Build history of the part. All positions in model axes, mm. Face numbers are marked on the shaded views. A direction names the side the tool comes from. Round coordinates to 2 decimals unless told otherwise and drop trailing zeros. Loops run counter-clockwise (first coordinate to the right, second up) from the corner with the lowest first, then second, coordinate; pieces in that order, holes last. Notation, with made-up numbers: M -27,4.25 L 0,4.25 A16 ccw 0,31.25 Z; hole C 63,-30.75 d8. An arc over 180 degrees is marked long. Use one line per item in the form item = value. Start each with the question number.
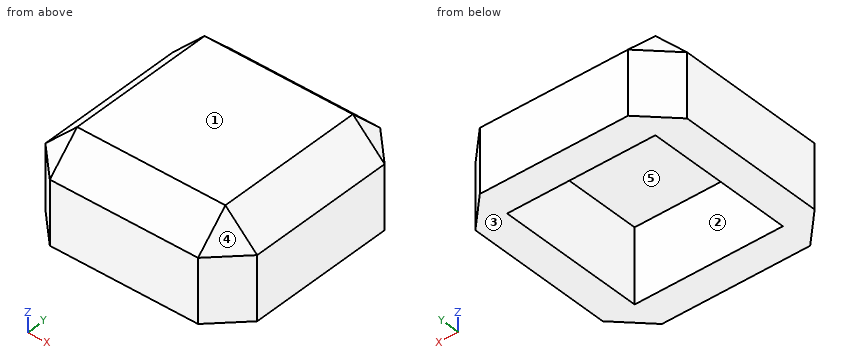
```python
from build123d import *

# Parameters (mm, degrees)
F0_W     = 10
F0_H     = 10
F0_W_2   = 7
F0_H_2   = 7
F1_DEPTH = 1
F2_DEPTH = 3.5
F3_SIZE  = 1.5


with BuildPart() as f1:
    # F0 (on Top) → F1 (new body)
    with BuildSketch(Plane.XY):
        Rectangle(F0_W, F0_H)
        Rectangle(F0_W_2, F0_H_2, mode=Mode.SUBTRACT)
        Rectangle(F0_W_2, F0_H_2)
    extrude(amount=F1_DEPTH)

    # F0 (on Top) → F2 (join)
    with BuildSketch(Plane.XY):
        Rectangle(F0_W, F0_H)
        Rectangle(F0_W_2, F0_H_2, mode=Mode.SUBTRACT)
    extrude(amount=-F2_DEPTH)

    # F3
    f3_edges = [f1.edges().sort_by_distance(p)[0] for p in [
        (5, -5, -1.25),
        (-5, -5, -1.25),
        (-5, 5, -1.25),
        (5, 5, -1.25),
        (0, -5, 1),
        (0, 5, 1),
        (-5, 0, 1),
        (5, 0, 1),
    ]]
    chamfer(f3_edges, length=F3_SIZE)


solid = f1.part
```
Q1. Saw through at B-B (z = 0.35). Give the cut face in (x, y), and give its area (3 significant figures).
Q2. Pull direction Z, two halves, no side cores. Call the marked faces 1, 2 and 3: pulls with the +Z half, pulls with the -Z half, needs draft (parallel to the pull), parting line crosses it, or undercut.
Q3. Tool access for the marked faces 4 and 5: list every direction of +Z, -Z, +X, -X, +Y, -Y with a clear straight run to the whole face (end or side of a thin tool).
Q4. Saw through at D-D (z = -1.05). Give the cut face in (x, y), and give its area (3 significant figures).
Q5. Saw through at C-C (x = 3.75). Give the cut face in (y, z).
Q6. Drop a flat-ended pin along its axis: P1, Ø1.5, axis at x = 1, y = 0, coming from the -Z side. Give the stop position or say it passes through.
Q7. Wall check: probe 1 along X at (y, z) = (0.25, -2.15); probe 2 along Z at (x, y) = (3.25, 2.5). Give the ranges that are in metal, low to high.
Q8. Saw through at A-A (y = 1). Give the cut face in (x, z).
Filled in:
q1.outline = M -4.15,-3.5 L -3.5,-4.15 L 3.5,-4.15 L 4.15,-3.5 L 4.15,3.5 L 3.5,4.15 L -3.5,4.15 L -4.15,3.5 Z
q1.area = 68.0 mm²
q2.face_1 = pulls with the +Z half
q2.face_2 = needs draft
q2.face_3 = pulls with the -Z half
q3.face_4 = +Z, +X, -Y
q3.face_5 = -Z
q4.outline = M -5,-3.5 L -3.5,-5 L 3.5,-5 L 5,-3.5 L 5,3.5 L 3.5,5 L -3.5,5 L -5,3.5 Z; hole M -3.5,-3.5 L 3.5,-3.5 L 3.5,3.5 L -3.5,3.5 Z
q4.area = 46.5 mm²
q5.outline = M -4.75,-3.5 L 4.75,-3.5 L 4.75,-0.5 L 3.5,0.75 L -3.5,0.75 L -4.75,-0.5 Z
q6.P1 = 0
q7.probe_1 = -5 to -3.5, 3.5 to 5
q7.probe_2 = 0 to 1
q8.outline = M -5,-3.5 L -3.5,-3.5 L -3.5,0 L 3.5,0 L 3.5,-3.5 L 5,-3.5 L 5,-0.5 L 3.5,1 L -3.5,1 L -5,-0.5 Z
